Geometry: final body of the model. Coordinates: model frame, mm. Face numbers are marked on the shaded views. Give positions to 0.01 mm unless a question says otherwise; leave off trailing zeros. Write each loop counter-clockwise with the first axis right and the second up, starting at its lowest first coordinate (ties: lowest second). Pieces come first, ordered by that corner, then holes. Notation, with made-up numbers: (9, -35) - (58, -35) arc R18 cw to (58, -23) - close; hole circle Ø10 at (26.5, 33). An arc over 180 degrees is marked (long way). Use CSV: the item, a comma, the result in double quotes. Start each with the question number.
(1) First-contact query: pin 1 Ø3 at (y, z) = (8.5, -14) entering from -X; pin 2 Ø2 at (x, y) = (15.5, 3) entering from +Z; pin 3 Ø4 at (x, y) = (2, 7) entering from -Z; pin 4 Ø4.5 at (x, z) = (20, -12.5) entering from -Y. Flat tips, straight axial feed; report the tip coordinate or a pass-through.
(2) Section C-C on y = 0.5. Output: boundary loops of the cut face in (x, z), and give its area (3 significant figures).
(3) Draft query along X for the marked faces 1, 2 and 3. Return one class per face: released by +X, released by -X, zero draft, split by the parting line, or undercut.
(4) Section B-B on x = 20. Output: boundary loops of the cut face in (y, z).
(5) Line query: probe 1 along Z at (x, y) = (20, 6); probe 2 along Z at (x, y) = (19, 5.75); probe 3 along Z at (x, y) = (-2.5, 6). Output: solid intervals per line, ascending. Write a range as [from, to].
(6) Section A-A on z = 0. Output: boundary loops of the cut face in (x, y).
(7) Section D-D on y = 8.75. Output: boundary loops of the cut face in (x, z).
from build123d import *

# Parameters (mm, degrees)
BOSS_EXTRUDE1_DEPTH  = 10
M5_CLEARANCE_HOLE1_D = 5.5
FILLET1_R            = 2


with BuildPart() as part:
    # Sketch1 → Boss-Extrude1 (new body)
    with BuildSketch(Plane(origin=(0, 0, 0), x_dir=(1, 0, 0), z_dir=(0, 1, 0))):
        with BuildLine():
            Line((-4.234491912, -6.190240564), (14.677005392, -19.126827043))
            ThreePointArc((14.677005392, -19.126827043), (16.022524994, -19.776721429), (17.5, -20))
            Line((17.5, -20), (22.5, -20))
            ThreePointArc((22.5, -20), (26.035533906, -18.535533906), (27.5, -15))
            Line((27.5, -15), (27.5, 15))
            ThreePointArc((27.5, 15), (26.035533906, 18.535533906), (22.5, 20))
            Line((22.5, 20), (17.5, 20))
            ThreePointArc((17.5, 20), (16.022524994, 19.776721429), (14.677005392, 19.126827043))
            Line((14.677005392, 19.126827043), (-4.234491912, 6.190240564))
            ThreePointArc((-4.234491912, 6.190240564), (-7.5, 0), (-4.234491912, -6.190240564))
        make_face()
    extrude(amount=BOSS_EXTRUDE1_DEPTH)

    # M5 Clearance Hole1 (through all)
    with Locations(Plane(origin=(0, 10, 0), x_dir=(1, 0, 0), z_dir=(0, 1, 0))):
        with Locations((0, 0), (20, 12.5), (20, -12.5)):
            Hole(M5_CLEARANCE_HOLE1_D / 2)

    # Fillet1
    fillet1_edges = [part.edges().sort_by_distance(p)[0] for p in [
        (16.022524994, 10, 19.776721429),
        (20, 10, 20),
        (26.035533906, 10, 18.535533906),
        (27.5, 10, 0),
        (26.035533906, 10, -18.535533906),
        (20, 10, -20),
        (16.022524994, 10, -19.776721429),
        (5.22125674, 10, -12.658533804),
        (-7.5, 10, 0),
        (5.22125674, 10, 12.658533804),
    ]]
    fillet(fillet1_edges, radius=FILLET1_R)


solid = part.part
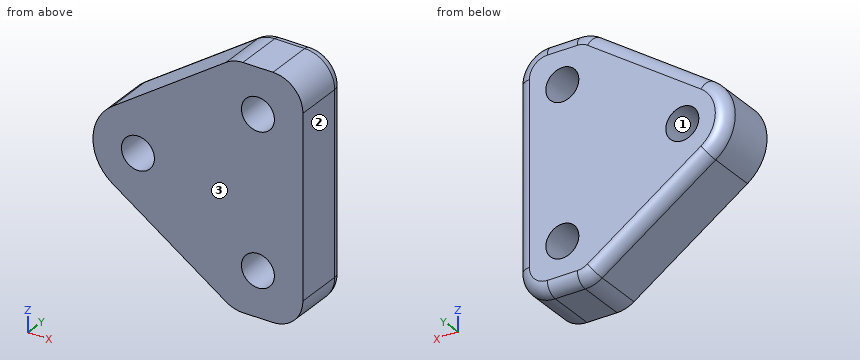
Check values:
1,pin 1,"stops at x = 5.05"
1,pin 2,"stops at z = 19.9"
1,pin 3,"stops at z = -11.82"
1,pin 4,"passes through"
2,outline,"(-4.23, -6.19) - (14.68, -19.13) arc R5 ccw to (17.5, -20) - (22.5, -20) arc R5 ccw to (27.5, -15) - (27.5, 15) arc R5 ccw to (22.5, 20) - (17.5, 20) arc R5 ccw to (14.68, 19.13) - (-4.23, 6.19) arc R7.5 ccw to start; hole circle Ø5.5 at (0, 0); hole circle Ø5.5 at (20, -12.5); hole circle Ø5.5 at (20, 12.5)"
2,area,"937 mm²"
3,face 1,"undercut"
3,face 2,"released by +X"
3,face 3,"zero draft"
4,outline,"(0, -20) - (8, -20) arc R2 ccw to (10, -18) - (10, -15.25) - (0, -15.25) - close; (0, -9.75) - (10, -9.75) - (10, 9.75) - (0, 9.75) - close; (0, 15.25) - (10, 15.25) - (10, 18) arc R2 ccw to (8, 20) - (0, 20) - close"
5,probe 1,"z = [-20, -15.25], [-9.75, 9.75], [15.25, 20]"
5,probe 2,"z = [-20, -15.06], [-9.94, 9.94], [15.06, 20]"
5,probe 3,"z = [-7.38, -1.15], [1.15, 7.38]"
6,outline,"(-7.5, 0) - (-2.75, 0) - (-2.75, 10) - (-5.5, 10) arc R2 ccw to (-7.5, 8) - close; (2.75, 0) - (27.5, 0) - (27.5, 8) arc R2 ccw to (25.5, 10) - (2.75, 10) - close"
7,outline,"(-4.15, -6.07) - (14.76, -19.01) arc R4.85 ccw to (17.5, -19.85) - (22.5, -19.85) arc R4.85 ccw to (27.35, -15) - (27.35, 15) arc R4.85 ccw to (22.5, 19.85) - (17.5, 19.85) arc R4.85 ccw to (14.76, 19.01) - (-4.15, 6.07) arc R7.35 ccw to start; hole circle Ø5.5 at (0, 0); hole circle Ø5.5 at (20, -12.5); hole circle Ø5.5 at (20, 12.5)"
